The model under review builds one solid part; all positions refer to its coordinate system, in mm. A direction names the side the tool comes from. Round coordinates to 2 decimals unless told otherwise and drop trailing zeros. Write each loop counter-clockwise with the first axis right and the second up, starting at its lowest first coordinate (ties: lowest second). Pieces come first, ordered by that corner, then holes. Notation, with made-up numbers: (-33.75, 13.5) -> (-15.75, 13.5) arc R24 ccw to (-15.75, 38.5) -> close; hole circle Ø4 at (71.5, -16.5). An arc over 180 degrees is marked (long way). Return JSON: item names as keys, results as strings. Group by question number.
1. Tool access review of faces 1 (the cylindrical face through (8.75, 6.99, 1.51)), 2 (the cylindrical face through (-13.36, 4.43, 1.48)), 3 (the flat face through (11, 9, 1)): name each direction out of +Z, -Z, +X, -X, +Y, -Y from which nothing blocks a thin tool from reaching the whole face with its end or side.
2. Mouldability with a two-part tool opening along Y and no side actions: class faces 4 (the cylindrical face through (-15.4, -4.49, 8.43)), 5 (the cylindrical face through (-10, 0, 1)), 6 (the flat face through (-13, 5, 2.499)) as pulls with the +Y half, pulls with the -Y half, needs draft (parallel to the pull), parting line crosses it, or undercut.
3. Take a section at B-B, the plane y = 0. Write out the cut boundary in (x, z) (3 decimals).
4. For line 1 along Y through (x, z) = (-13, 1.55) (3 decimals); line 2 along Y through (x, z) = (7, 8.5); line 3 along Y through (x, z) = (1, 4.25), list the stretches that pass through material, from the lowest coordinate up. Write a range as from..to.
5. Take a section at A-A, the plane z = 5.5. Write out the cut boundary in (x, y), then the cut area to 3 significant figures.
6. Clearance check with flat-ended pins moving along their axes: P1, Ø4.5, axis at x = -1.5, y = 4.5, coming from the -Z side; P2, Ø4, axis at x = 0.5, y = 8.5, coming from the +Z side; P3, Ø0.8, axis at y = 7, z = 0.5, coming from the +X side. State where each tip first meets the part, or that it passes through.
from build123d import *

# Parameters (mm, degrees)
BOSS_EXTRUDE1_DEPTH     = 2
SKETCH2_R               = 1.575
BOSS_EXTRUDE2_DEPTH     = 4
SKETCH3_R               = 1.8
BOSS_EXTRUDE3_DEPTH     = 0.75
SKETCH4_W               = 2
SKETCH4_H               = 17
BOSS_EXTRUDE4_DEPTH     = 0.001
SKETCH5_W               = 18
SKETCH5_H               = 2
BOSS_EXTRUDE5_DEPTH     = 0.001
SKETCH6_W               = 2.001
SKETCH6_H               = 2
BOSS_EXTRUDE6_DEPTH     = 5
BOSS_EXTRUDE7_DEPTH     = 0.001
CUT_EXTRUDE1_DEPTH      = 20.519323784
SKETCH9_W               = 2.937742252
SKETCH9_H               = 8
CUT_EXTRUDE2_DEPTH      = 0.001
CUT_EXTRUDE11_START     = -0.001
SKETCH21_R              = 9.75
SKETCH21_R_2            = 1.8
CUT_EXTRUDE11_DEPTH     = 0.001
SKETCH10_W              = 32
SKETCH10_H              = 2
BOSS_EXTRUDE8_DEPTH     = 7
FILLET1_R               = 0.5
SKETCH11_R              = 0.625
BOSS_EXTRUDE9_DEPTH     = 2
SKETCH14_W              = 2
SKETCH14_H              = 2
CUT_EXTRUDE5_DEPTH      = 22.401355237
SKETCH12_R              = 0.675
CUT_EXTRUDE3_DEPTH      = 2.5
CUT_EXTRUDE6_DEPTH      = 2
FILLET2_R               = 0.5
FILLET3_R               = 0.5
FILLET4_R               = 2
CUT_EXTRUDE7_DEPTH      = 26.019992106
CUT_EXTRUDE7_DEPTH_BACK = 1
SKETCH19_R              = 0.625
CUT_EXTRUDE9_DEPTH      = 2


with BuildPart() as part:
    # Sketch1 → Boss-Extrude1 (new body)
    with BuildSketch(Plane.XY):
        Polygon((-11, 6), (-11, 11), (11, 11), (11, 6), (11, -6), (-11, -6), align=None)
    extrude(amount=BOSS_EXTRUDE1_DEPTH)

    # Sketch3 → Boss-Extrude3 (add)
    with BuildSketch(Plane(origin=(0, 0, 0), x_dir=(-1, 0, 0), z_dir=(0, 0, -1))):
        with Locations(Location((0, 0, 0), (0, 0, 180))):
            Circle(SKETCH3_R)
    extrude(amount=BOSS_EXTRUDE3_DEPTH)

    # Sketch4 → Boss-Extrude4 (add)
    with BuildSketch(Plane(origin=(0, 0, 0), x_dir=(-1, 0, 0), z_dir=(0, 0, -1))):
        with Locations((10, 2.5)):
            Rectangle(SKETCH4_W, SKETCH4_H)
        with Locations((-10, 2.5)):
            Rectangle(SKETCH4_W, SKETCH4_H)
    extrude(amount=BOSS_EXTRUDE4_DEPTH)

    # Sketch5 → Boss-Extrude5 (add)
    with BuildSketch(Plane(origin=(0, 0, 0), x_dir=(-1, 0, 0), z_dir=(0, 0, -1))):
        with Locations((0, 10)):
            Rectangle(SKETCH5_W, SKETCH5_H)
    extrude(amount=BOSS_EXTRUDE5_DEPTH)

    # Sketch6 → Boss-Extrude6 (add)
    with BuildSketch(Plane(origin=(11, 0, 0), x_dir=(0, 0, -1), z_dir=(1, 0, 0))):
        with Locations((-0.9995, -5)):
            Rectangle(SKETCH6_W, SKETCH6_H)
        with Locations((-0.9995, 5)):
            Rectangle(SKETCH6_W, SKETCH6_H)
    boss_extrude6 = extrude(amount=BOSS_EXTRUDE6_DEPTH)

    # Mirror1: Boss-Extrude6 across plane
    add(boss_extrude6.mirror(Plane(origin=(0, 0, 0), x_dir=(0, 0, 1), z_dir=(1, 0, 0))))

    # Sketch7 → Boss-Extrude7 (add)
    with BuildSketch(Plane(origin=(0, 0, -0.001), x_dir=(-1, 0, 0), z_dir=(0, 0, -1))):
        with BuildLine():
            ThreePointArc((-6.708203932, -6), (-8.407551231, -3.211398808), (-9, 0))
            Line((-9, 0), (-9, -6))
            Line((-9, -6), (-6.708203932, -6))
        make_face()
        with BuildLine():
            Line((-9, 9), (-9, 0))
            ThreePointArc((-9, 0), (-6.363961031, 6.363961031), (0, 9))
            Line((0, 9), (-9, 9))
        make_face()
    boss_extrude7 = extrude(amount=-BOSS_EXTRUDE7_DEPTH)

    # Sketch8 → Cut-Extrude1 (cut, through all)
    with BuildSketch(Plane(origin=(0, 0, -0.001), x_dir=(-1, 0, 0), z_dir=(0, 0, -1))):
        with BuildLine():
            Line((-11, 4), (-9.16515139, 4))
            ThreePointArc((-9.16515139, 4), (-10, 0), (-9.16515139, -4))
            Line((-9.16515139, -4), (-11, -4))
            Line((-11, -4), (-11, 4))
        make_face()
    cut_extrude1 = extrude(amount=-CUT_EXTRUDE1_DEPTH, mode=Mode.SUBTRACT)

    # Sketch9 → Cut-Extrude2 (cut)
    with BuildSketch(Plane(origin=(0, 0, -0.001), x_dir=(-1, 0, 0), z_dir=(0, 0, -1))):
        with Locations((-9.531128874, 0)):
            Rectangle(SKETCH9_W, SKETCH9_H)
    cut_extrude2 = extrude(amount=-CUT_EXTRUDE2_DEPTH, mode=Mode.SUBTRACT)

    # Mirror2: Boss-Extrude7, Cut-Extrude1, Cut-Extrude2 across plane
    add(boss_extrude7.mirror(Plane(origin=(0, 0, 0), x_dir=(0, 0, 1), z_dir=(1, 0, 0))))
    add(cut_extrude1.mirror(Plane(origin=(0, 0, 0), x_dir=(0, 0, 1), z_dir=(1, 0, 0))), mode=Mode.SUBTRACT)
    add(cut_extrude2.mirror(Plane(origin=(0, 0, 0), x_dir=(0, 0, 1), z_dir=(1, 0, 0))), mode=Mode.SUBTRACT)

    # Sketch21 → Cut-Extrude11 (cut)
    with BuildSketch(Plane(origin=(0, 0, -0.001), x_dir=(-1, 0, 0), z_dir=(0, 0, -1)).offset(CUT_EXTRUDE11_START)):
        Circle(SKETCH21_R)
        with Locations(Location((0, 0, 0), (0, 0, 180))):
            Circle(SKETCH21_R_2, mode=Mode.SUBTRACT)
    extrude(amount=CUT_EXTRUDE11_DEPTH, mode=Mode.SUBTRACT)

    # Sketch10 → Boss-Extrude8 (add)
    with BuildSketch(Plane.XY.offset(2)):
        with Locations((0, -5)):
            Rectangle(SKETCH10_W, SKETCH10_H)
        with Locations((0, 5)):
            Rectangle(SKETCH10_W, SKETCH10_H)
    extrude(amount=BOSS_EXTRUDE8_DEPTH)

    # Fillet1
    fillet1_edges = [part.edges().sort_by_distance(p)[0] for p in [
        (10, 0, 2),
        (-10, 0, 2),
    ]]
    fillet(fillet1_edges, radius=FILLET1_R)

    # Sketch11 → Boss-Extrude9 (add)
    with BuildSketch(Plane(origin=(0, 0, -0.001), x_dir=(-1, 0, 0), z_dir=(0, 0, -1))):
        with Locations(Location((-13, -5, 0), (0, 0, 180))):
            Circle(SKETCH11_R)
    boss_extrude9 = extrude(amount=BOSS_EXTRUDE9_DEPTH)

    # Sketch14 → Cut-Extrude5 (cut, through all)
    with BuildSketch(Plane(origin=(0, 0, -0.001), x_dir=(-1, 0, 0), z_dir=(0, 0, -1))):
        with Locations((10, 7)):
            Rectangle(SKETCH14_W, SKETCH14_H)
        with Locations((-10, 7)):
            Rectangle(SKETCH14_W, SKETCH14_H)
    extrude(amount=-CUT_EXTRUDE5_DEPTH, mode=Mode.SUBTRACT)

    # Sketch12 → Cut-Extrude3 (cut)
    with BuildSketch(Plane(origin=(0, 0, -0.001), x_dir=(-1, 0, 0), z_dir=(0, 0, -1))):
        with Locations((13, -5)):
            Circle(SKETCH12_R)
    cut_extrude3 = extrude(amount=-CUT_EXTRUDE3_DEPTH, mode=Mode.SUBTRACT)

    # Sketch16 → Cut-Extrude6 (cut)
    with BuildSketch(Plane(origin=(0, 6, 0), x_dir=(1, 0, 0), z_dir=(0, 1, 0))):
        with BuildLine():
            Line((-9, -1), (-9, -2))
            ThreePointArc((-9, -2), (-8.75, -1.5), (-9, -1))
        make_face()
    cut_extrude6 = extrude(amount=CUT_EXTRUDE6_DEPTH, mode=Mode.SUBTRACT)

    # Mirror3: Boss-Extrude9, Cut-Extrude3 across plane
    add(boss_extrude9.mirror(Plane.ZX))
    add(cut_extrude3.mirror(Plane.ZX), mode=Mode.SUBTRACT)

    # Mirror4: Cut-Extrude6 across plane
    add(cut_extrude6.mirror(Plane(origin=(0, 0, 0), x_dir=(0, 0, 1), z_dir=(1, 0, 0))), mode=Mode.SUBTRACT)

    # Fillet2
    fillet2_edges = [part.edges().sort_by_distance(p)[0] for p in [
        (12.375, -5, -0.001),
        (12.375, 5, -0.001),
    ]]
    fillet(fillet2_edges, radius=FILLET2_R)

    # Fillet3
    # the kernel refuses this fillet: 0.5 mm, written as the material it takes off along each edge
    with BuildSketch(Plane(origin=(-13, -5, -0.001), x_dir=(-1, 0, 0), z_dir=(0, -1, 0))) as fillet3_piece_1:
        with BuildLine():
            CenterArc((0.675 + FILLET3_R, -FILLET3_R), FILLET3_R, 90, 90)
            Line((0.675, -FILLET3_R), (0.675, 0))
            Line((0.675, 0), (0.675 + FILLET3_R, 0))
        make_face()
    revolve(axis=Axis((-13, -5, -0.001), (0, 0, -1)), mode=Mode.SUBTRACT)
    with BuildSketch(Plane(origin=(-13, 5, -0.001), x_dir=(-1, 0, 0), z_dir=(0, 1, 0))) as fillet3_piece_2:
        with BuildLine():
            CenterArc((0.675 + FILLET3_R, FILLET3_R), FILLET3_R, 180, 90)
            Line((0.675, FILLET3_R), (0.675, 0))
            Line((0.675, 0), (0.675 + FILLET3_R, 0))
        make_face()
    revolve(axis=Axis((-13, 5, -0.001), (0, 0, 1)), mode=Mode.SUBTRACT)

    # Fillet4
    fillet4_edges = [part.edges().sort_by_distance(p)[0] for p in [
        (16, -5, 9),
        (-16, -5, 9),
        (-16, 5, 9),
        (16, 5, 9),
    ]]
    fillet(fillet4_edges, radius=FILLET4_R)

    # Sketch17 → Cut-Extrude7 (cut, two sides: drawn at the far end of the back side and taken through both)
    with BuildSketch(Plane.XZ.offset(6).offset(-CUT_EXTRUDE7_DEPTH_BACK)):
        with BuildLine():
            Line((-16, 7), (-16, -0.001))
            Line((-16, -0.001), (-14.5, -0.001))
            Line((-14.5, -0.001), (-14.5, 7))
            ThreePointArc((-14.5, 7), (-14.353553391, 7.353553391), (-14, 7.5))
            Line((-14, 7.5), (14, 7.5))
            ThreePointArc((14, 7.5), (14.353553391, 7.353553391), (14.5, 7))
            Line((14.5, 7), (14.5, -0.001))
            Line((14.5, -0.001), (16, -0.001))
            Line((16, -0.001), (16, 7))
            ThreePointArc((16, 7), (15.414213562, 8.414213562), (14, 9))
            Line((14, 9), (-14, 9))
            ThreePointArc((-14, 9), (-15.414213562, 8.414213562), (-16, 7))
        make_face()
    extrude(amount=CUT_EXTRUDE7_DEPTH + CUT_EXTRUDE7_DEPTH_BACK, mode=Mode.SUBTRACT)

    # Sketch19 → Cut-Extrude9 (cut)
    with BuildSketch(Plane(origin=(0, 6, 0), x_dir=(1, 0, 0), z_dir=(0, 1, 0))):
        with Locations(Location((0, -2.625, 0), (0, 0, 90))):
            Circle(SKETCH19_R)
        with Locations(Location((0, -8.125, 0), (0, 0, 270))):
            Circle(SKETCH19_R)
    extrude(amount=-CUT_EXTRUDE9_DEPTH, mode=Mode.SUBTRACT)


with BuildPart() as body_2:
    # Sketch2 → Boss-Extrude2 (new body)
    with BuildSketch(Plane(origin=(0, 0, 2), x_dir=(-1, 0, 0), z_dir=(0, 0, -1))):
        Circle(SKETCH2_R)
    extrude(amount=BOSS_EXTRUDE2_DEPTH)


with BuildPart() as part_1:
    add(part.part)

    # Combine2: cut body 2
    add(body_2.part, mode=Mode.SUBTRACT)


solid = part_1.part
Output:
{
 "1": {"face 1": "+X", "face 2": "-Z", "face 3": "+Z, -Z, +X, +Y"},
 "2": {"face 4": "needs draft", "face 5": "undercut", "face 6": "undercut"},
 "3": {"outline": "(-10, 0) -> (-1.8, 0) -> (-1.8, -0.75) -> (-1.575, -0.75) -> (-1.575, 2) -> (-9.5, 2) arc R0.5 ccw to (-10, 1.5) -> close; (1.575, -0.75) -> (1.8, -0.75) -> (1.8, 0) -> (10, 0) -> (10, 1.5) arc R0.5 ccw to (9.5, 2) -> (1.575, 2) -> close"},
 "4": {"line 1": "y = -6..-5.675, -4.325..-4, 4..4.325, 5.675..6", "line 2": "y = -5..-4, 4..6", "line 3": "y = -6..-4, 4..6"},
 "5": {"outline": "(-16, -5) -> (-14.5, -5) -> (-14.5, -6) -> (14.5, -6) -> (14.5, -5) -> (16, -5) -> (16, -4) -> (-16, -4) -> close; (-16, 4) -> (16, 4) -> (16, 6) -> (-16, 6) -> close", "area": "125 mm^2"},
 "6": {"P1": "stops at z = 0", "P2": "stops at z = 2", "P3": "stops at x = 9"}
}
